```python
from build123d import *

# Parameters (mm, degrees)
SKETCH_1_W                          = 77
SKETCH_1_H                          = 106
TRAY_FLOOR_1_DEPTH                  = 2
SKETCH_2_W                          = 3
SKETCH_2_H                          = 106
LEFT_RETAINER_2_DEPTH               = 10.5
SKETCH_3_W                          = 3
SKETCH_3_H                          = 106
RIGHT_RETAINER_3_DEPTH              = 10.5
SKETCH_4_W                          = 71
SKETCH_4_H                          = 3.5
FRONT_RETAINER_4_DEPTH              = 10.5
SKETCH_5_W                          = 22
SKETCH_5_H                          = 8
PULL_HANDLE_5_DEPTH                 = 4
SKETCH_6_W                          = 3
SKETCH_6_H                          = 5
LEFT_EAR_BRIDGE_6_DEPTH             = 10
SKETCH_7_W                          = 3
SKETCH_7_H                          = 5
RIGHT_EAR_BRIDGE_7_DEPTH            = 10
SKETCH_8_W                          = 9.5
SKETCH_8_H                          = 3.5
LEFT_LOCK_EAR_8_DEPTH               = 10
SKETCH_9_W                          = 9.5
SKETCH_9_H                          = 3
RIGHT_LOCK_EAR_9_DEPTH              = 10
SKETCH_10_R                         = 1.7
TRAY_LOCK_M3_CLEARANCE_10_DEPTH     = 5
SKETCH_11_W                         = 48
SKETCH_11_H                         = 9
TRAY_AIRFLOW_11_DEPTH               = 4
SKETCH_12_R                         = 1.65
DRIVE_SIDE_M3_12_DEPTH              = 80
SKETCH_13_W                         = 14
SKETCH_13_H                         = 3
HANDLE_GRIP_13_DEPTH                = 6
SKETCH_14_W                         = 7.5
SKETCH_14_H                         = 4.2
LEFT_FLANGE_CLEARANCE_1_DEPTH       = 15
SKETCH_16_W                         = 3.3
SKETCH_16_H                         = 7
FRONT_ADJUSTABLE_M3_SLOT_1_DEPTH    = 80
SKETCH_17_W                         = 3.3
SKETCH_17_H                         = 7
REAR_ADJUSTABLE_M3_SLOT_2_DEPTH     = 80
SKETCH_18_W                         = 62
SKETCH_18_H                         = 3.2
SATA_PLUG_LOWER_CLEARANCE_301_DEPTH = 5


with BuildPart() as part:
    # Эскиз1 → Tray_floor_1 (new body)
    with BuildSketch(Plane.XY):
        with Locations((0, -9)):
            Rectangle(SKETCH_1_W, SKETCH_1_H)
    extrude(amount=TRAY_FLOOR_1_DEPTH)

    # Эскиз2 → Left_retainer_2 (add)
    with BuildSketch(Plane.XY.offset(2)):
        with Locations((-37, -9)):
            Rectangle(SKETCH_2_W, SKETCH_2_H)
    extrude(amount=LEFT_RETAINER_2_DEPTH)

    # Эскиз3 → Right_retainer_3 (add)
    with BuildSketch(Plane.XY.offset(2)):
        with Locations((37, -9)):
            Rectangle(SKETCH_3_W, SKETCH_3_H)
    extrude(amount=RIGHT_RETAINER_3_DEPTH)

    # Эскиз4 → Front_retainer_4 (add)
    with BuildSketch(Plane.XY.offset(2)):
        with Locations((0, -60.25)):
            Rectangle(SKETCH_4_W, SKETCH_4_H)
    extrude(amount=FRONT_RETAINER_4_DEPTH)

    # Эскиз5 → Pull_handle_5 (add)
    with BuildSketch(Plane.XY):
        with Locations((0, -66)):
            Rectangle(SKETCH_5_W, SKETCH_5_H)
    extrude(amount=PULL_HANDLE_5_DEPTH)

    # Эскиз6 → Left_ear_bridge_6 (add)
    with BuildSketch(Plane.XY):
        with Locations((-37, -62.5)):
            Rectangle(SKETCH_6_W, SKETCH_6_H)
    extrude(amount=LEFT_EAR_BRIDGE_6_DEPTH)

    # Эскиз7 → Right_ear_bridge_7 (add)
    with BuildSketch(Plane.XY):
        with Locations((37, -62.5)):
            Rectangle(SKETCH_7_W, SKETCH_7_H)
    extrude(amount=RIGHT_EAR_BRIDGE_7_DEPTH)

    # Эскиз8 → Left_lock_ear_8 (add)
    with BuildSketch(Plane.XY):
        with Locations((-40.25, -65.25)):
            Rectangle(SKETCH_8_W, SKETCH_8_H)
    extrude(amount=LEFT_LOCK_EAR_8_DEPTH)

    # Эскиз9 → Right_lock_ear_9 (add)
    with BuildSketch(Plane.XY):
        with Locations((40.25, -65.5)):
            Rectangle(SKETCH_9_W, SKETCH_9_H)
    extrude(amount=RIGHT_LOCK_EAR_9_DEPTH)

    # Эскиз10 → Tray_lock_M3_clearance_10 (cut)
    with BuildSketch(Plane(origin=(0, -68, 0), x_dir=(1, 0, 0), z_dir=(0, 1, 0))):
        with Locations(Location((-41, -5, 0), (0, 0, 90))):
            Circle(SKETCH_10_R)
        with Locations(Location((41, -5, 0), (0, 0, 90))):
            Circle(SKETCH_10_R)
    extrude(amount=TRAY_LOCK_M3_CLEARANCE_10_DEPTH, mode=Mode.SUBTRACT)

    # Эскиз11 → Tray_airflow_11 (cut)
    with BuildSketch(Plane.XY.offset(-1)):
        with Locations((0, -40.5)):
            Rectangle(SKETCH_11_W, SKETCH_11_H)
        with Locations((0, -23.5)):
            Rectangle(SKETCH_11_W, SKETCH_11_H)
        with Locations((0, -6.5)):
            Rectangle(SKETCH_11_W, SKETCH_11_H)
        with Locations((0, 10.5)):
            Rectangle(SKETCH_11_W, SKETCH_11_H)
        with Locations((0, 27.5)):
            Rectangle(SKETCH_11_W, SKETCH_11_H)
    extrude(amount=TRAY_AIRFLOW_11_DEPTH, mode=Mode.SUBTRACT)

    # Эскиз12 → Drive_side_M3_12 (cut)
    with BuildSketch(Plane(origin=(-40, 0, 0), x_dir=(0, 0, -1), z_dir=(1, 0, 0))):
        with Locations(Location((-5, -45.55, 0), (0, 0, 180))):
            Circle(SKETCH_12_R)
        with Locations(Location((-5, 31.05, 0), (0, 0, 180))):
            Circle(SKETCH_12_R)
    extrude(amount=DRIVE_SIDE_M3_12_DEPTH, mode=Mode.SUBTRACT)

    # Эскиз13 → Handle_grip_13 (cut)
    with BuildSketch(Plane.XY.offset(-1)):
        with Locations((0, -66.5)):
            Rectangle(SKETCH_13_W, SKETCH_13_H)
    extrude(amount=HANDLE_GRIP_13_DEPTH, mode=Mode.SUBTRACT)

    # Эскиз14 → Left_flange_clearance_1 (cut)
    with BuildSketch(Plane.XY.offset(-1)):
        with Locations((-42.25, -62.1)):
            Rectangle(SKETCH_14_W, SKETCH_14_H)
    extrude(amount=LEFT_FLANGE_CLEARANCE_1_DEPTH, mode=Mode.SUBTRACT)

    # Эскиз16 → Front_adjustable_M3_slot_1 (cut)
    with BuildSketch(Plane(origin=(-40, 0, 0), x_dir=(0, 0, -1), z_dir=(1, 0, 0))):
        with Locations((-5, -44.5)):
            Rectangle(SKETCH_16_W, SKETCH_16_H)
    extrude(amount=FRONT_ADJUSTABLE_M3_SLOT_1_DEPTH, mode=Mode.SUBTRACT)

    # Эскиз17 → Rear_adjustable_M3_slot_2 (cut)
    with BuildSketch(Plane(origin=(-40, 0, 0), x_dir=(0, 0, -1), z_dir=(1, 0, 0))):
        with Locations((-5, 31.5)):
            Rectangle(SKETCH_17_W, SKETCH_17_H)
    extrude(amount=REAR_ADJUSTABLE_M3_SLOT_2_DEPTH, mode=Mode.SUBTRACT)

    # Эскиз18 → SATA_plug_lower_clearance_301 (cut)
    with BuildSketch(Plane.XY.offset(-1)):
        with Locations((0, 43.4)):
            Rectangle(SKETCH_18_W, SKETCH_18_H)
    extrude(amount=SATA_PLUG_LOWER_CLEARANCE_301_DEPTH, mode=Mode.SUBTRACT)


solid = part.part
```
Verification items for the finished model (mm, model axes). A direction names the side the tool comes from. Coordinates: 2 decimals unless noted, no trailing zeros. Loops run counter-clockwise (first coordinate to the right, second up) from the corner with the lowest first, then second, coordinate; pieces in that order, holes last. Notation, with made-up numbers: (32.25, 3) -> (79.25, 3) arc R20 ccw to (79.25, 32) -> close; hole circle Ø5 at (16.25, 4.25). An arc over 180 degrees is marked (long way). Answer in a Markdown table with one row per item. Add a question column.
1. Access from +Z, -Z, +X, -X, +Y, -Y to the whole of each face (thin tool, end or side, straight path). Record for faces 1 (the face through (-43, -64.2, 4)), 2 (the face through (0, -64, 4)), 3 (the face through (37, -45, 3.35)).
2. Material ranges on probe 1 along X at (y, z) = (-66.15, 5); probe 2 along X at (y, z) = (-54, 10.25); probe 3 along Y at (x, z) = (-27, 8), recorded low to high. Write a range as [from, to].
3. Section check C-C, the plane y = 7.5. Enter the section's corners in (x, z), then the cut area to 3 significant figures.
4. Depth check by flat-ended pin: P1, Ø2, axis at y = -7.5, z = 7.5, coming from the +X side; P2, Ø1.6, axis at x = -3, z = 0.5, coming from the +Y side; P3, Ø2, axis at x = 27.5, z = 6, coming from the +Y side. Enter the tip coordinate at first touch or a pass-through.
5. Draft check along Y on faces 4 (the face through (39, -67, 5)), 5 (the face through (-38.5, -11, 6)), 6 (the face through (37, -41, 5)). Enter one of: +Y half, -Y half, draft (parallel to the pull), parting line (faces both ways), or undercut.
6. Section check A-A, the plane x = -41. Enter the section's corners in (y, z), then the cut area to 3 significant figures.
7. Section check D-D, the plane z = 11.25. Enter the section's corners in (x, y), then the cut area to 4 significant figures.
8. Section check B-B, the plane x = -21.5. Enter the section's corners in (y, z).
Derived:
| question | item | result |
|---|---|---|
| 1 | face 1 | +Z, -Z, -X, +Y |
| 1 | face 2 | +Z, -Y |
| 1 | face 3 | +X, -X |
| 2 | probe 1 | x = [-45, -42.7], [-39.3, -35.5], [35.5, 39.3], [42.7, 45] |
| 2 | probe 2 | x = [-38.5, -35.5], [35.5, 38.5] |
| 2 | probe 3 | y = [-62, -58.5] |
| 3 | outline | (-38.5, 0) -> (-24, 0) -> (-24, 2) -> (-35.5, 2) -> (-35.5, 12.5) -> (-38.5, 12.5) -> close; (24, 0) -> (38.5, 0) -> (38.5, 12.5) -> (35.5, 12.5) -> (35.5, 2) -> (24, 2) -> close |
| 3 | area | 121 mm² |
| 4 | P1 | stops at x = 38.5 |
| 4 | P2 | stops at y = 41.8 |
| 4 | P3 | stops at y = -58.5 |
| 5 | face 4 | -Y half |
| 5 | face 5 | draft |
| 5 | face 6 | undercut |
| 6 | outline | (-67, 0) -> (-64.2, 0) -> (-64.2, 3.3) -> (-67, 3.3) -> close; (-67, 6.7) -> (-64.2, 6.7) -> (-64.2, 10) -> (-67, 10) -> close |
| 6 | area | 18.5 mm² |
| 7 | outline | (-38.5, -62) -> (38.5, -62) -> (38.5, 44) -> (35.5, 44) -> (35.5, -58.5) -> (-35.5, -58.5) -> (-35.5, 44) -> (-38.5, 44) -> close |
| 7 | area | 884.5 mm² |
| 8 | outline | (-62, 0) -> (-45, 0) -> (-45, 2) -> (-58.5, 2) -> (-58.5, 12.5) -> (-62, 12.5) -> close; (-36, 0) -> (-28, 0) -> (-28, 2) -> (-36, 2) -> close; (-19, 0) -> (-11, 0) -> (-11, 2) -> (-19, 2) -> close; (-2, 0) -> (6, 0) -> (6, 2) -> (-2, 2) -> close; (15, 0) -> (23, 0) -> (23, 2) -> (15, 2) -> close; (32, 0) -> (41.8, 0) -> (41.8, 2) -> (32, 2) -> close |
